Build history of the part. All positions in model axes, mm. A direction names the side the tool comes from. Round coordinates to 2 decimals unless told otherwise and drop trailing zeros. Write each loop counter-clockwise with the first axis right and the second up, starting at its lowest first coordinate (ties: lowest second). Pieces come first, ordered by that corner, then holes.
1) Saw through at D-D (x = -19). Write the cut outline in (y, z).
2) Saw through at B-B (y = -4.5). Write the cut outline in (x, z).
3) Wall check: probe 1 along X at (y, z) = (-12, -7); probe 2 along Z at (x, y) = (31, -12.5); probe 3 along Y at (x, z) = (10.5, -1.5). Give the ranges that are in metal, low to high.
4) Saw through at C-C (z = -5). Write the cut outline in (x, y).
5) Flat gauge pins, fed straight in: pin 1 (6 mm diameter, centred on x = -8, z = -8.5, fed in from +Y); pin 2 (3.5 mm diameter, centred on x = -0.5, y = -32, fed in from +Z); pin 3 (3 mm diameter, centred on x = -9.5, z = -2, fed in from +Y). Where does each tip first touch, or does it go through?
6) Pull direction X, two halves, no side cores. Call faces 1 (the flat face through (-37.75, -17, -5)), 2 (the cylindrical face through (0.1, -13, -3.5)), 3 (the flat face through (-27, 0, -3)): +X half, -X half, draft (parallel to the pull), parting line (faces both ways), or undercut.
7) Which spindle directions (+Z, -Z, +X, -X, +Y, -Y) get a long thin tool onto all of the face, cutting with end or side? Do faces 4 (the flat face through (-15.5, -1, -2)), 5 (the flat face through (20, -15, -4)), 6 (the flat face through (-7, -25, -2)). Say none if no direction does.
8) Saw through at A-A (x = 0). Write the cut outline in (y, z).
from build123d import *

# Parameters (mm, degrees)
F1_DEPTH = 31
F3_DEPTH = 3
F5_DEPTH = 4
F7_DEPTH = 3.2
F9_DEPTH = 7


with BuildPart() as f1:
    # F0 (on Front) → F1 (new body)
    with BuildSketch(Plane.XZ):
        Polygon((37.75, 0), (-37.75, 0), (-37.75, -10), (-34.75, -10), (-34.75, -4), (-5, -4), (-5, -3.8), (5, -3.8), (5, -4), (34.75, -4), (34.75, -10), (37.75, -10), align=None)
    extrude(amount=F1_DEPTH)

    # F2 (on face) → F3 (join)
    with BuildSketch(Plane.XZ.offset(31)):
        Polygon((37.75, 0), (-37.75, 0), (-37.75, -10), (-34.75, -10), (-34.75, -4), (-5, -4), (-5, -3.8), (5, -3.8), (5, -4), (34.75, -4), (34.75, -10), (37.75, -10), align=None)
        Polygon((-34.75, -4), (-34.75, -10), (34.75, -10), (34.75, -4), (5, -4), (5, -3.8), (-5, -3.8), (-5, -4), align=None)
    extrude(amount=F3_DEPTH)

    # F4 (on face) → F5 (cut)
    with BuildSketch(Plane.XY):
        with BuildLine():
            Line((-4, -17), (-4, -34))
            Line((-4, -34), (4, -34))
            Line((4, -34), (4, -17))
            ThreePointArc((4, -17), (0, -13), (-4, -17))
        make_face()
        Polygon((15.5, 0), (-15.5, 0), (-15.5, -3), (-5, -3), (-5, -8), (5, -8), (5, -3), (15.5, -3), align=None)
    extrude(amount=-F5_DEPTH, mode=Mode.SUBTRACT)

    # F6 (on face) → F7 (cut)
    with BuildSketch(Plane.XY):
        with BuildLine():
            Line((-7, -17), (-7, -34))
            Line((-7, -34), (-4, -34))
            Line((-4, -34), (-4, -17))
            ThreePointArc((-4, -17), (0, -13), (4, -17))
            Line((4, -17), (4, -34))
            Line((4, -34), (7, -34))
            Line((7, -34), (7, -17))
            ThreePointArc((7, -17), (0, -10), (-7, -17))
        make_face()
    extrude(amount=-F7_DEPTH, mode=Mode.SUBTRACT)

    # F8 (on face) → F9 (cut)
    with BuildSketch(Plane(origin=(0, 0, -10), x_dir=(1, 0, 0), z_dir=(0, 0, -1))):
        with BuildLine():
            Line((-34.75, 31), (-32.75, 31))
            ThreePointArc((-32.75, 31), (-36.1642135624, 32.4142135624), (-34.75, 29))
            Line((-34.75, 29), (-34.75, 31))
        make_face()
        with BuildLine():
            ThreePointArc((-34.75, 29), (-33.3357864376, 29.5857864376), (-32.75, 31))
            Line((-32.75, 31), (-34.75, 31))
            Line((-34.75, 31), (-34.75, 29))
        make_face()
        with BuildLine():
            ThreePointArc((36.75, 31), (34.75, 33), (32.75, 31))
            Line((32.75, 31), (34.75, 31))
            Line((34.75, 31), (34.75, 29))
            ThreePointArc((34.75, 29), (36.1642135624, 29.5857864376), (36.75, 31))
        make_face()
        with BuildLine():
            Line((34.75, 31), (32.75, 31))
            ThreePointArc((32.75, 31), (33.3357864376, 29.5857864376), (34.75, 29))
            Line((34.75, 29), (34.75, 31))
        make_face()
    extrude(amount=-F9_DEPTH, mode=Mode.SUBTRACT)


solid = f1.part
Evaluation:
1. outline: (-34, -10) - (-31, -10) - (-31, -4) - (0, -4) - (0, 0) - (-34, 0) - close
2. outline: (-37.75, -10) - (-34.75, -10) - (-34.75, -4) - (-5, -4) - (-5, 0) - (-37.75, 0) - close; (5, -4) - (34.75, -4) - (34.75, -10) - (37.75, -10) - (37.75, 0) - (5, 0) - close
3. probe 1: x = -37.75 to -34.75, 34.75 to 37.75
3. probe 2: z = -4 to 0
3. probe 3: y = -34 to -3
4. outline: (-37.75, -34) - (37.75, -34) - (37.75, 0) - (34.75, 0) - (34.75, -29) arc R2 cw (long way) to (32.75, -31) - (-32.75, -31) arc R2 cw (long way) to (-34.75, -29) - (-34.75, 0) - (-37.75, 0) - close
5. pin 1: stops at y = -31
5. pin 2: stops at z = -4
5. pin 3: stops at y = -3
6. face 1: -X half
6. face 2: undercut
6. face 3: draft
7. face 4: +Z, -Z, +Y
7. face 5: -Z, +Y
7. face 6: +Z, -Y
8. outline: (-34, -10) - (-31, -10) - (-31, -4) - (-34, -4) - close; (-13, -3.8) - (-8, -3.8) - (-8, 0) - (-10, 0) - (-10, -3.2) - (-13, -3.2) - close
